from build123d import *

# Parameters (mm, degrees)
ESQUISSE1_R        = 3.625
BOSS_EXTRU_1_DEPTH = 40
CONG_1_R           = 1
CONG_2_R           = 1


with BuildPart() as part:
    # Esquisse1 → Boss.-Extru.1 (new body)
    with BuildSketch(Plane(origin=(0, 0, 0), x_dir=(1, 0, 0), z_dir=(0, 1, 0))):
        with Locations(Location((0, 0, 0), (0, 0, 270))):
            Circle(ESQUISSE1_R)
    extrude(amount=BOSS_EXTRU_1_DEPTH)

    # Congé1
    cong_1_edges = [part.edges().sort_by_distance(p)[0] for p in [
        (0, 40, -3.625),
    ]]
    fillet(cong_1_edges, radius=CONG_1_R)

    # Congé2
    cong_2_edges = [part.edges().sort_by_distance(p)[0] for p in [
        (0, 0, -3.625),
    ]]
    fillet(cong_2_edges, radius=CONG_2_R)


solid = part.part
Design review of the part built by this model. Coordinates are the model's own, in mm. Give positions to 0.01 mm unless a question says otherwise; leave off trailing zeros. Write each loop counter-clockwise with the first axis right and the second up, starting at its lowest first coordinate (ties: lowest second). Pieces come first, ordered by that corner, then holes. Notation, with made-up numbers: M 7,-24 L 44,-24 A23 ccw 44,-10 Z; hole C 71.25,-25 d9. An arc over 180 degrees is marked long. Return JSON: item names as keys, results as strings. Group by question number.
Item 1: Take a section at A-A (y = 11). Give the boundary of the cut face in (x, z) (3 decimals).
Item 2: Clearance check with flat-ended pins moving along their axes: pin 1 Ø4 at (y, z) = (19, -3) entering from +X; pin 2 Ø1 at (x, y) = (-2.5, 21) entering from +Z. State where each tip first meets the part, or that it passes through.
Item 3: Wall thickness on line 1 along Z through (x, y) = (2.5, 31.5) (3 decimals); line 2 along X through (y, z) = (4, -0.25): over which ranges is each line inside the solid? List them lowest first.
Return value:
{
 "1": {"outline": "C 0,0 d7.25"},
 "2": {"pin 1": "stops at x = 3.48", "pin 2": "stops at z = 3.02"},
 "3": {"line 1": "z = -2.625 to 2.625", "line 2": "x = -3.62 to 3.62"}
}
